from build123d import *

# Parameters (mm, degrees)
F0_R           = 50.216863
F1_DEPTH       = 25.4
F2_R           = 2.54
F3_R           = 2.54
F4_D           = 6.35
F4_CBORE_D     = 12.7
F4_CBORE_DEPTH = 6.35


with BuildPart() as f1:
    # F0 (on Top) → F1 (new body)
    with BuildSketch(Plane.XY):
        Circle(F0_R)
    extrude(amount=F1_DEPTH)

    # F2
    f2_edges = [f1.edges().sort_by_distance(p)[0] for p in [
        (-50.216863, 0, 25.4),
    ]]
    fillet(f2_edges, radius=F2_R)

    # F3
    f3_edges = [f1.edges().sort_by_distance(p)[0] for p in [
        (-50.216863, 0, 0),
    ]]
    fillet(f3_edges, radius=F3_R)

    # F4 (through all)
    with Locations(Plane(origin=(0, 0, 0), x_dir=(1, 0, 0), z_dir=(0, 0, -1))):
        with Locations((0, 0)):
            CounterBoreHole(F4_D / 2, F4_CBORE_D / 2, F4_CBORE_DEPTH)


solid = f1.part
Geometry check sheet. Reference: the model listing, model coordinates, mm. A direction names the side the tool comes from. Give positions to 0.01 mm unless a question says otherwise; leave off trailing zeros. Loops run counter-clockwise (first coordinate to the right, second up) from the corner with the lowest first, then second, coordinate; pieces in that order, holes last.
(1) Set-up check for faces 4 (the flat face through (-2, -3, 6.35)), 5 (the cylindrical face through (0.69, 3.1, 16.01)): record each of +Z, -Z, +X, -X, +Y, -Y from which the full face is reachable in a straight line by a thin tool's end or side.
From the geometry:
face 4: -Z
face 5: +Z, -Z
(2) Depth check by flat-ended pin: pin 1 Ø4 at (x, y) = (0.5, 3) entering from -Z; pin 2 Ø3 at (x, z) = (-18.5, 9.5) entering from -Y; pin 3 Ø1.5 at (y, z) = (4.5, 8.5) entering from -X; pin 4 Ø12 at (x, y) = (-37, 22) entering from -Z. Enter the tip coordinate at first touch or a pass-through.
From the geometry:
pin 1: stops at z = 6.35
pin 2: stops at y = -47.25
pin 3: stops at x = -50.08
pin 4: stops at z = 0
(3) Thickness scan on L1, parallel to Y at x = 0, z = 15.5 (3 decimals); L2, parallel to Y at x = 33, z = 23.25; L3, parallel to Y at x = 28, z = 8.5. Record the ranges inside material, lowest first.
From the geometry:
L1: y = -50.217 to -3.175, 3.175 to 50.217
L2: y = -37.81 to 37.81
L3: y = -41.69 to 41.69
(4) Section check C-C on z = 5. Record the cut outline in (x, y), then the cut area to 3 significant figures.
From the geometry:
outline: circle Ø100.43 at (0, 0); hole circle Ø12.7 at (0, 0)
area: 7,800 mm2
(5) Release check for a two-part mould opening along X. For faces 1 (the cylindrical face through (47.9, 15.08, 12.56)), 2 (the cylindrical face through (-1.38, 6.2, 3.13)), 3 (the flat face through (-1, -10, 0)) record: released by +X, released by -X, zero draft, split by the parting line, or undercut.
From the geometry:
face 1: split by the parting line
face 2: undercut
face 3: zero draft
(6) Section check A-A on y = 0. Record the cut outline in (x, z) (3 decimals).
From the geometry:
outline: (-50.217, 2.54) arc R2.54 ccw to (-47.677, 0) - (-6.35, 0) - (-6.35, 6.35) - (-3.175, 6.35) - (-3.175, 25.4) - (-47.677, 25.4) arc R2.54 ccw to (-50.217, 22.86) - close; (3.175, 6.35) - (6.35, 6.35) - (6.35, 0) - (47.677, 0) arc R2.54 ccw to (50.217, 2.54) - (50.217, 22.86) arc R2.54 ccw to (47.677, 25.4) - (3.175, 25.4) - close
